from build123d import *

# Parameters (mm, degrees)
BOSS_EXTRUDE1_DEPTH = 85
SKETCH3_R           = 1.5
CUT_EXTRUDE2_DEPTH  = 129.44162098
CUT_EXTRUDE3_DEPTH  = 99.07777526
SKETCH5_W           = 90
SKETCH5_H           = 8
BOSS_EXTRUDE2_DEPTH = 3
SKETCH6_R           = 1.5
CUT_EXTRUDE4_DEPTH  = 99.07777526
FILLET4_R           = 6
FILLET5_R           = 7.5
CUT_EXTRUDE5_DEPTH  = 129.44162098


with BuildPart() as part:
    # Sketch1 → Boss-Extrude1 (new body)
    with BuildSketch(Plane.XY):
        Polygon((-45, 0), (45, 0), (45, -7.5), (48, -7.5), (48, 2), (-48, 2), (-48, -7.5), (-45, -7.5), align=None)
    extrude(amount=BOSS_EXTRUDE1_DEPTH)

    # Sketch3 → Cut-Extrude2 (cut, through all)
    with BuildSketch(Plane.ZY.offset(48)):
        with Locations(Location((25, -3, 0), (0, 0, 270))):
            Circle(SKETCH3_R)
        with Locations(Location((60, -3, 0), (0, 0, 270))):
            Circle(SKETCH3_R)
    extrude(amount=-CUT_EXTRUDE2_DEPTH, mode=Mode.SUBTRACT)

    # Sketch4 → Cut-Extrude3 (cut, through all)
    with BuildSketch(Plane(origin=(0, 2, 0), x_dir=(1, 0, 0), z_dir=(0, 1, 0))):
        with BuildLine():
            Line((-37.5, -53.5), (-37.5, -66.5))
            ThreePointArc((-37.5, -66.5), (-41.25, -70.25), (-45, -66.5))
            Line((-45, -66.5), (-45, -53.5))
            ThreePointArc((-45, -53.5), (-41.25, -49.75), (-37.5, -53.5))
        make_face()
        with BuildLine():
            Line((-45, -18.5), (-45, -31.5))
            ThreePointArc((-45, -31.5), (-41.25, -35.25), (-37.5, -31.5))
            Line((-37.5, -31.5), (-37.5, -18.5))
            ThreePointArc((-37.5, -18.5), (-41.25, -14.75), (-45, -18.5))
        make_face()
        with BuildLine():
            Line((45, -31.5), (45, -18.5))
            ThreePointArc((45, -18.5), (41.25, -14.75), (37.5, -18.5))
            Line((37.5, -18.5), (37.5, -31.5))
            ThreePointArc((37.5, -31.5), (41.25, -35.25), (45, -31.5))
        make_face()
        with BuildLine():
            Line((45, -66.5), (45, -53.5))
            ThreePointArc((45, -53.5), (41.25, -49.75), (37.5, -53.5))
            Line((37.5, -53.5), (37.5, -66.5))
            ThreePointArc((37.5, -66.5), (41.25, -70.25), (45, -66.5))
        make_face()
    extrude(amount=-CUT_EXTRUDE3_DEPTH, mode=Mode.SUBTRACT)

    # Sketch5 → Boss-Extrude2 (add)
    with BuildSketch(Plane.XZ):
        with Locations((0, 81)):
            Rectangle(SKETCH5_W, SKETCH5_H)
        with Locations((0, 4)):
            Rectangle(SKETCH5_W, SKETCH5_H)
    extrude(amount=BOSS_EXTRUDE2_DEPTH)

    # Sketch6 → Cut-Extrude4 (cut, through all)
    with BuildSketch(Plane(origin=(0, 2, 0), x_dir=(1, 0, 0), z_dir=(0, 1, 0))):
        with Locations(Location((-17.5, -4, 0), (0, 0, 180))):
            Circle(SKETCH6_R)
        with Locations(Location((17.5, -4, 0), (0, 0, 180))):
            Circle(SKETCH6_R)
        with Locations(Location((-17.5, -81, 0), (0, 0, 180))):
            Circle(SKETCH6_R)
        with Locations(Location((17.5, -81, 0), (0, 0, 180))):
            Circle(SKETCH6_R)
        with Locations(Location((-10, -4, 0), (0, 0, 180))):
            Circle(SKETCH6_R)
        with Locations(Location((10, -4, 0), (0, 0, 180))):
            Circle(SKETCH6_R)
        with Locations(Location((-10, -81, 0), (0, 0, 180))):
            Circle(SKETCH6_R)
        with Locations(Location((10, -81, 0), (0, 0, 180))):
            Circle(SKETCH6_R)
    extrude(amount=-CUT_EXTRUDE4_DEPTH, mode=Mode.SUBTRACT)

    # Fillet4
    fillet4_edges = [part.edges().sort_by_distance(p)[0] for p in [
        (-45, -1.5, 77),
        (45, -1.5, 77),
        (-45, -1.5, 8),
        (45, -1.5, 8),
    ]]
    fillet(fillet4_edges, radius=FILLET4_R)

    # Fillet5
    fillet5_edges = [part.edges().sort_by_distance(p)[0] for p in [
        (45, 0, 42.5),
        (-45, 0, 42.5),
    ]]
    fillet(fillet5_edges, radius=FILLET5_R - 0.0001)  # a hair under: the kernel refuses the full size

    # Sketch7 → Cut-Extrude5 (cut, through all)
    with BuildSketch(Plane(origin=(48, 0, 0), x_dir=(0, 0, -1), z_dir=(1, 0, 0))):
        Polygon((-75, -3), (-85, -3), (-85, -7.5), (-70.5, -7.5), align=None)
        Polygon((-10, -3), (-14.5, -7.5), (0, -7.5), (0, -3), align=None)
    extrude(amount=-CUT_EXTRUDE5_DEPTH, mode=Mode.SUBTRACT)


solid = part.part
Geometry check sheet. Reference: the model listing, model coordinates, mm. A direction names the side the tool comes from. Round coordinates to 2 decimals unless told otherwise and drop trailing zeros. Write each loop counter-clockwise with the first axis right and the second up, starting at its lowest first coordinate (ties: lowest second). Pieces come first, ordered by that corner, then holes. Notation, with made-up numbers: (-23, -27) - (15, -27) arc R11 cw to (15, -23) - close; hole circle Ø4 at (7, 31.5). An arc over 180 degrees is marked (long way). One line per item, written item: value.
1. Cross-section at A-A on x = -17.5. Record the boundary of the cut face in (y, z), and give its area (3 significant figures).
The answers:
outline: (-3, 0) - (2, 0) - (2, 2.5) - (-3, 2.5) - close; (-3, 5.5) - (2, 5.5) - (2, 79.5) - (-3, 79.5) - (-3, 77) - (0, 77) - (0, 8) - (-3, 8) - close; (-3, 82.5) - (2, 82.5) - (2, 85) - (-3, 85) - close
area: 188 mm^2
2. Cross-section at B-B on z = 4. Record the boundary of the cut face in (x, y), and give its area (3 significant figures).
The answers:
outline: (-48, -3) - (-19, -3) - (-19, 2) - (-48, 2) - close; (-16, -3) - (-11.5, -3) - (-11.5, 2) - (-16, 2) - close; (-8.5, -3) - (8.5, -3) - (8.5, 2) - (-8.5, 2) - close; (11.5, -3) - (16, -3) - (16, 2) - (11.5, 2) - close; (19, -3) - (48, -3) - (48, 2) - (19, 2) - close
area: 420 mm^2
3. Depth check by flat-ended pin: pin 1 Ø1.8 at (y, z) = (-3, 60) entering from -X; pin 2 Ø15.5 at (x, z) = (19, 75.5) entering from -Y; pin 3 Ø2 at (x, z) = (-28.5, 48.5) entering from -Y. Enter the tip coordinate at first touch or a pass-through.
The answers:
pin 1: passes through
pin 2: stops at y = -3
pin 3: stops at y = 0
4. Cross-section at D-D on x = 35. Record the boundary of the cut face in (y, z), and give its area (3 significant figures).
The answers:
outline: (-3, 0) - (2, 0) - (2, 85) - (-3, 85) - (-3, 77) - (0, 77) - (0, 8) - (-3, 8) - close
area: 218 mm^2
5. Scan lines: L1, parallel to Z at x = -10, y = -1.4; L2, parallel to X at y = 1.75, z = 66; L3, parallel to Z at x = -35, y = -1. Record each from-to range of solid material in increasing order.
The answers:
L1: z = 0 to 2.5, 5.5 to 8, 77 to 79.5, 82.5 to 85
L2: x = -48 to -45, -37.5 to 37.5, 45 to 48
L3: z = 0 to 8, 77 to 85
6. Mould release check, pull along Z, two halves, no side actions. Record for faces 1 (the face through (46, -7.5, 42)), 2 (the face through (-46, -5, 12)), 3 (the face through (37.5, 1, 60)): released by +Z, released by -Z, zero draft, split by the parting line, or undercut.
The answers:
face 1: zero draft
face 2: released by -Z
face 3: undercut
7. Set-up check for faces 4 (the face through (-45, -3, 56)), 5 (the face through (47, -5, 12)), 6 (the face through (-37.5, 1, 60)): record each of +Z, -Z, +X, -X, +Y, -Y from which the full face is reachable in a straight line by a thin tool's end or side.
The answers:
face 4: -Y
face 5: -Z, +X, -X, -Y
face 6: +Y, -Y
